Model file for the job. Use its own axes, mm. A direction names the side the tool comes from. Round coordinates to 2 decimals unless told otherwise and drop trailing zeros. Loops run counter-clockwise (first coordinate to the right, second up) from the corner with the lowest first, then second, coordinate; pieces in that order, holes last. Notation, with made-up numbers: M 44,-34.5 L 87,-34.5 A35 cw 87,2.5 Z; hole C 89,-14 d6. An arc over 180 degrees is marked long. Answer in a Markdown table with one row per item.
from build123d import *

# Parameters (mm, degrees)
SKETCH_1_R        = 1.75
EXTRUDE_1_DEPTH   = 5.8
SKETCH_2_R        = 2.75
SKETCH_2_R_2      = 1.75
EXTRUDE_1_2_DEPTH = 1.5


with BuildPart() as part:
    # 草图1 → Extrude 1 (new body)
    with BuildSketch(Plane.XZ.offset(8.55)):
        with Locations(Location((24.091410852, -9.546220913, 0), (0, 0, 270))):
            Circle(SKETCH_1_R)
    extrude(amount=EXTRUDE_1_DEPTH)

    # 草图2 → Extrude 1 2 (add)
    with BuildSketch(Plane(origin=(0, -10.25, 0), x_dir=(1, 0, 0), z_dir=(0, 1, 0))):
        with Locations((24.091410852, 9.546220913)):
            Circle(SKETCH_2_R)
        with Locations((24.091410852, 9.546220913)):
            Circle(SKETCH_2_R_2, mode=Mode.SUBTRACT)
    extrude(amount=-EXTRUDE_1_2_DEPTH)


solid = part.part
1. Saw through at B-B (x = 23.05). Write the cut outline in (y, z), and give its area (3 significant figures).
Verdict:
| item | result |
|---|---|
| outline | M -14.35,-10.95 L -11.75,-10.95 L -11.75,-12.09 L -10.25,-12.09 L -10.25,-10.95 L -8.55,-10.95 L -8.55,-8.14 L -10.25,-8.14 L -10.25,-7 L -11.75,-7 L -11.75,-8.14 L -14.35,-8.14 Z |
| area | 19.7 mm² |
2. Wall check: probe 1 along Y at (x, z) = (23.3, -11.4); probe 2 along X at (y, z) = (-12.9, -9.6); probe 3 along X at (y, z) = (-10.7, -9.45). Give the ranges that are in metal, low to high.
Verdict:
| item | result |
|---|---|
| probe 1 | y = -11.75 to -10.25 |
| probe 2 | x = 22.34 to 25.84 |
| probe 3 | x = 21.34 to 26.84 |
3. Saw through at D-D (x = 21.9). Write the cut outline in (y, z), and give its area (3 significant figures).
Verdict:
| item | result |
|---|---|
| outline | M -11.75,-11.21 L -10.25,-11.21 L -10.25,-7.88 L -11.75,-7.88 Z |
| area | 4.98 mm² |
4. Pin check, flat tips, straight feed: pin 1 (1 mm diameter, centred on x = 23, y = -12, fed in from -Z); pin 2 (2 mm diameter, centred on y = -13.5, z = -11.5, fed in from -X). Stop position of each tip, or through.
Verdict:
| item | result |
|---|---|
| pin 1 | stops at z = -12.22 |
| pin 2 | stops at x = 22.62 |
5. Saw through at A-A (z = -10.8). Write the cut outline in (x, y).
Verdict:
| item | result |
|---|---|
| outline | M 21.64,-11.75 L 22.87,-11.75 L 22.87,-14.35 L 25.31,-14.35 L 25.31,-11.75 L 26.54,-11.75 L 26.54,-10.25 L 25.31,-10.25 L 25.31,-8.55 L 22.87,-8.55 L 22.87,-10.25 L 21.64,-10.25 Z |
6. Saw through at C-C (y = -9.6). Write the cut outline in (x, z).
Verdict:
| item | result |
|---|---|
| outline | C 24.09,-9.55 d3.5 |
7. Tool access for faces 1 (the flat face through (26, -11.75, -10)), 2 (the flat face through (24, -14.35, -10)), 3 (the flat face through (26, -10.25, -10)): list every direction of +Z, -Z, +X, -X, +Y, -Y with a clear straight run to the whole face (end or side of a thin tool).
Verdict:
| item | result |
|---|---|
| face 1 | -Y |
| face 2 | +Z, -Z, +X, -X, -Y |
| face 3 | +Y |
